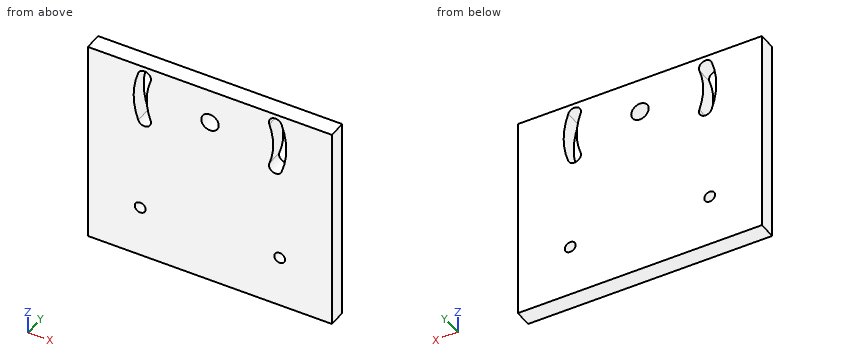
from build123d import *

# Parameters (mm, degrees)
F0_W     = 184.15
F0_H     = 152.4
F0_R     = 6.35
F1_DEPTH = 12.7
F3_DEPTH = 12.701
F6_D     = 7.9375


with BuildPart() as f1:
    # F0 (on Front) → F1 (new body)
    with BuildSketch(Plane.XZ):
        with Locations((-3.175, -50.8)):
            Rectangle(F0_W, F0_H)
        Circle(F0_R, mode=Mode.SUBTRACT)
    extrude(amount=F1_DEPTH)

    # F2 (on face) → F3 (cut, through all)
    with BuildSketch(Plane.XZ.offset(12.7)):
        with BuildLine():
            ThreePointArc((52.211671, -19.003494), (55.5625, 0), (52.211671, 19.003494))
            ThreePointArc((52.211671, 19.003494), (46.107514, 21.849909), (43.261099, 15.745752))
            ThreePointArc((43.261099, 15.745752), (46.0375, 0), (43.261099, -15.745752))
            ThreePointArc((43.261099, -15.745752), (46.107514, -21.849909), (52.211671, -19.003494))
        make_face()
    extrude(amount=-F3_DEPTH, mode=Mode.SUBTRACT)

    # F4: F1 across plane


with BuildPart() as f1_1:
    add(f1.part)
    add(f1.part.mirror(Plane.YZ), mode=Mode.INTERSECT)

    # F6 (through all)
    with Locations(Plane.XZ.offset(12.7)):
        with Locations((50.8, -88.9), (-50.8, -88.9)):
            Hole(F6_D / 2)


solid = f1_1.part
The model under review builds one solid part; all positions refer to its coordinate system, in mm. Round coordinates to 2 decimals unless told otherwise and drop trailing zeros. Loops run counter-clockwise (first coordinate to the right, second up) from the corner with the lowest first, then second, coordinate; pieces in that order, holes last. Notation, with made-up numbers: (68.5, 45) -> (108.5, 45) arc R20 cw to (108.5, 67) -> close; hole circle Ø11 at (-7.75, -22.5). An arc over 180 degrees is marked (long way). One line per question, with ' | ' between items. Start each with the question number.
Item 1: Add section B-B, the plane y = -6.5. Count the separate pieces of the cut face and the enclosed holes in it, then the cut area to 3 significant figures.
Item 2: For pin 1 (7 mm diameter, centred on x = -50.8, z = -88.9, fed in from +Y), flat-tipped, find the tip position at first contact; note if it passes through.
Item 3: Add section A-A, the plane z = 0. Write out the cut boundary in (x, y), then the cut area to 3 significant figures.
Item 4: Add section C-C, the plane x = 0. Write out the cut boundary in (y, z).
Item 5: Add section D-D, the plane z = -88.9. Write out the cut boundary in (x, y), then the cut area to 3 significant figures.
Item 6: Wall thickness on line 1 along X through (y, z) = (-8.5, 0); line 2 along Z through (x, y) = (50.8, -7.25); line 3 along Z through (x, y) = (0, -5): over which ranges is each line inside the solid? List them lowest first. Write a range as [from, to].
Return value:
1) separate pieces: 1 | enclosed holes: 5 | area: 26,100 mm2
2) pin 1: passes through
3) outline: (-88.9, -12.7) -> (-55.56, -12.7) -> (-55.56, 0) -> (-88.9, 0) -> close; (-46.04, -12.7) -> (-6.35, -12.7) -> (-6.35, 0) -> (-46.04, 0) -> close; (6.35, -12.7) -> (46.04, -12.7) -> (46.04, 0) -> (6.35, 0) -> close; (55.56, -12.7) -> (88.9, -12.7) -> (88.9, 0) -> (55.56, 0) -> close | area: 1,850 mm2
4) outline: (-12.7, -127) -> (0, -127) -> (0, -6.35) -> (-12.7, -6.35) -> close; (-12.7, 6.35) -> (0, 6.35) -> (0, 25.4) -> (-12.7, 25.4) -> close
5) outline: (-88.9, -12.7) -> (-54.77, -12.7) -> (-54.77, 0) -> (-88.9, 0) -> close; (-46.83, -12.7) -> (46.83, -12.7) -> (46.83, 0) -> (-46.83, 0) -> close; (54.77, -12.7) -> (88.9, -12.7) -> (88.9, 0) -> (54.77, 0) -> close | area: 2,060 mm2
6) line 1: x = [-88.9, -55.56], [-46.04, -6.35], [6.35, 46.04], [55.56, 88.9] | line 2: z = [-127, -92.87], [-84.93, -21.02], [21.02, 25.4] | line 3: z = [-127, -6.35], [6.35, 25.4]
